Geometry: final body of the model. Coordinates: model frame, mm. A direction names the side the tool comes from. Give positions to 0.01 mm unless a question says otherwise; leave off trailing zeros. Order: outer loops, then holes, each group sorted by start corner. A loop starts at its lowest first (then second) coordinate and runs counter-clockwise, first axis right, second up. Notation, with made-up numbers: (26.25, 21) -> (50.25, 21) arc R35 cw to (50.25, 57) -> close; hole circle Ø8 at (-11, -34.75). An arc over 180 degrees is marked (long way). Write item = value, one per line.
```python
from build123d import *

# Parameters (mm, degrees)
CYLINDER049_R           = 0.8
CYLINDER049_DEPTH       = 10
CYLINDER048_R           = 0.8
CYLINDER048_DEPTH       = 10
CYLINDER017_R           = 1
CYLINDER017_DEPTH       = 10
CYLINDER017_ROLL_ANGLE  = 90
CYLINDER011_R           = 2
CYLINDER011_DEPTH       = 10
CYLINDER011_PITCH_ANGLE = 90
CYLINDER014_R           = 2
CYLINDER014_DEPTH       = 10
CYLINDER014_PITCH_ANGLE = 90
CYLINDER013_R           = 2
CYLINDER013_DEPTH       = 10
CYLINDER013_PITCH_ANGLE = 90
CYLINDER015_R           = 2
CYLINDER015_DEPTH       = 10
CYLINDER015_PITCH_ANGLE = 90
CYLINDER002_W           = 14
CYLINDER002_H           = 8
CYLINDER002_ANGLE       = 180
CYLINDER001_W           = 15
CYLINDER001_H           = 10
CYLINDER001_ANGLE       = 180
CYLINDER003_W           = 14
CYLINDER003_H           = 8
CYLINDER003_ANGLE       = 180
CYLINDER_W              = 15
CYLINDER_H              = 10
CYLINDER_ANGLE          = 180
BOX001_W                = 28
BOX001_H                = 21
BOX001_DEPTH            = 8
BOX_W                   = 30
BOX_H                   = 21
BOX_DEPTH               = 10
FUSION_PLACEMENT_ANGLE  = 180
BOX014_W                = 28
BOX014_H                = 3
BOX014_DEPTH            = 3
BOX007_W                = 30
BOX007_H                = 3
BOX007_DEPTH            = 1


with BuildPart() as cilindro049:
    # Cylinder049 → Cylinder049 (new body)
    with BuildSketch(Plane(origin=(11, -17, -15), x_dir=(1, 0, 0), z_dir=(0, 0, 1))):
        Circle(CYLINDER049_R)
    extrude(amount=CYLINDER049_DEPTH)


with BuildPart() as cilindro048:
    # Cylinder048 → Cylinder048 (new body)
    with BuildSketch(Plane(origin=(11, -4, -15), x_dir=(1, 0, 0), z_dir=(0, 0, 1))):
        Circle(CYLINDER048_R)
    extrude(amount=CYLINDER048_DEPTH)


with BuildPart() as cilindro017:
    # Cylinder017 → Cylinder017 (new body)
    with BuildSketch(Plane.XY):
        Circle(CYLINDER017_R)
    extrude(amount=CYLINDER017_DEPTH)


with BuildPart() as cilindro017_1:
    # Cylinder017 roll: moved
    add(cilindro017.part.rotate(Axis((0, 0, 0), (1, 0, 0)), CYLINDER017_ROLL_ANGLE))


with BuildPart() as cilindro017_2:
    # Cylinder017 placement: moved
    add(cilindro017_1.part.moved(Location((-14, 90, 38.5))))


with BuildPart() as cilindro011:
    # Cylinder011 → Cylinder011 (new body)
    with BuildSketch(Plane.XY):
        Circle(CYLINDER011_R)
    extrude(amount=CYLINDER011_DEPTH)


with BuildPart() as cilindro011_1:
    # Cylinder011 pitch: moved
    add(cilindro011.part.rotate(Axis((0, 0, 0), (0, 1, 0)), CYLINDER011_PITCH_ANGLE))


with BuildPart() as cilindro011_2:
    # Cylinder011 placement: moved
    add(cilindro011_1.part.moved(Location((-32, 72.5, 39.5))))


with BuildPart() as cilindro014:
    # Cylinder014 → Cylinder014 (new body)
    with BuildSketch(Plane.XY):
        Circle(CYLINDER014_R)
    extrude(amount=CYLINDER014_DEPTH)


with BuildPart() as cilindro014_1:
    # Cylinder014 pitch: moved
    add(cilindro014.part.rotate(Axis((0, 0, 0), (0, 1, 0)), CYLINDER014_PITCH_ANGLE))


with BuildPart() as cilindro014_2:
    # Cylinder014 placement: moved
    add(cilindro014_1.part.moved(Location((-5, 46.5, 39.5))))


with BuildPart() as cilindro013:
    # Cylinder013 → Cylinder013 (new body)
    with BuildSketch(Plane.XY):
        Circle(CYLINDER013_R)
    extrude(amount=CYLINDER013_DEPTH)


with BuildPart() as cilindro013_1:
    # Cylinder013 pitch: moved
    add(cilindro013.part.rotate(Axis((0, 0, 0), (0, 1, 0)), CYLINDER013_PITCH_ANGLE))


with BuildPart() as cilindro013_2:
    # Cylinder013 placement: moved
    add(cilindro013_1.part.moved(Location((-32, 46.5, 39.5))))


with BuildPart() as cilindro015:
    # Cylinder015 → Cylinder015 (new body)
    with BuildSketch(Plane.XY):
        Circle(CYLINDER015_R)
    extrude(amount=CYLINDER015_DEPTH)


with BuildPart() as cilindro015_1:
    # Cylinder015 pitch: moved
    add(cilindro015.part.rotate(Axis((0, 0, 0), (0, 1, 0)), CYLINDER015_PITCH_ANGLE))


with BuildPart() as cilindro015_2:
    # Cylinder015 placement: moved
    add(cilindro015_1.part.moved(Location((-5, 72.5, 39.5))))


with BuildPart() as cilindro002:
    # Cylinder002 → Cylinder002 (revolve)
    with BuildSketch(Plane(origin=(16, 49, -36), x_dir=(1, 0, 0), z_dir=(0, 1, 0))):
        with Locations((7, 4)):
            Rectangle(CYLINDER002_W, CYLINDER002_H)
    revolve(axis=Axis((16, 49, -36), (0, 0, -1)), revolution_arc=CYLINDER002_ANGLE)


with BuildPart() as cut001:
    # Cylinder001 → Cylinder001 (revolve)
    with BuildSketch(Plane(origin=(16, 49, -34), x_dir=(1, 0, 0), z_dir=(0, 1, 0))):
        with Locations((7.5, 5)):
            Rectangle(CYLINDER001_W, CYLINDER001_H)
    revolve(axis=Axis((16, 49, -34), (0, 0, -1)), revolution_arc=CYLINDER001_ANGLE)

    # Cut001: cut Cilindro002
    add(cilindro002.part, mode=Mode.SUBTRACT)


with BuildPart() as cut001_1:
    # Cut001 placement: moved
    add(cut001.part.moved(Location((-3, 0, 0))))


with BuildPart() as cilindro003:
    # Cylinder003 → Cylinder003 (revolve)
    with BuildSketch(Plane(origin=(13, 70, -36), x_dir=(-1, 0, 0), z_dir=(0, -1, 0))):
        with Locations((7, 4)):
            Rectangle(CYLINDER003_W, CYLINDER003_H)
    revolve(axis=Axis((13, 70, -36), (0, 0, -1)), revolution_arc=CYLINDER003_ANGLE)


with BuildPart() as cut002:
    # Cylinder → Cylinder (revolve)
    with BuildSketch(Plane(origin=(13, 70, -34), x_dir=(-1, 0, 0), z_dir=(0, -1, 0))):
        with Locations((7.5, 5)):
            Rectangle(CYLINDER_W, CYLINDER_H)
    revolve(axis=Axis((13, 70, -34), (0, 0, -1)), revolution_arc=CYLINDER_ANGLE)

    # Cut002: cut Cilindro003
    add(cilindro003.part, mode=Mode.SUBTRACT)


with BuildPart() as cubo001:
    # Box001 → Box001 (new body)
    with BuildSketch(Plane(origin=(-1, 49, -44), x_dir=(1, 0, 0), z_dir=(0, 0, 1))):
        with Locations((14, 10.5)):
            Rectangle(BOX001_W, BOX001_H)
    extrude(amount=BOX001_DEPTH)


with BuildPart() as cut025:
    # Box → Box (new body)
    with BuildSketch(Plane(origin=(-2, 49, -44), x_dir=(1, 0, 0), z_dir=(0, 0, 1))):
        with Locations((15, 10.5)):
            Rectangle(BOX_W, BOX_H)
    extrude(amount=BOX_DEPTH)

    # Cut: cut Cubo001
    add(cubo001.part, mode=Mode.SUBTRACT)

    # Fusion: union Cut001, Cut002
    add(cut001_1.part)
    add(cut002.part)


with BuildPart() as cut025_1:
    # Fusion placement: moved
    add(cut025.part.rotate(Axis((0, 0, 0), (0, 1, 0)), FUSION_PLACEMENT_ANGLE))

    # Cut021: cut Cilindro015
    add(cilindro015_2.part, mode=Mode.SUBTRACT)

    # Cut022: cut Cilindro013
    add(cilindro013_2.part, mode=Mode.SUBTRACT)

    # Cut023: cut Cilindro014
    add(cilindro014_2.part, mode=Mode.SUBTRACT)

    # Cut024: cut Cilindro011
    add(cilindro011_2.part, mode=Mode.SUBTRACT)

    # Cut025: cut Cilindro017
    add(cilindro017_2.part, mode=Mode.SUBTRACT)


with BuildPart() as cubo014:
    # Box014 → Box014 (new body)
    with BuildSketch(Plane(origin=(-27, 58, 41), x_dir=(1, 0, 0), z_dir=(0, 0, 1))):
        with Locations((14, 1.5)):
            Rectangle(BOX014_W, BOX014_H)
    extrude(amount=BOX014_DEPTH)


with BuildPart() as cut068:
    # Box007 → Box007 (new body)
    with BuildSketch(Plane(origin=(-28, 58, 44), x_dir=(1, 0, 0), z_dir=(0, 0, 1))):
        with Locations((15, 1.5)):
            Rectangle(BOX007_W, BOX007_H)
    extrude(amount=BOX007_DEPTH)

    # Fusion002010: union Cubo014
    add(cubo014.part)

    # Fusion002015: union Cut025
    add(cut025_1.part)


with BuildPart() as cut068_1:
    # Fusion002015 placement: moved
    add(cut068.part.moved(Location((13, -70, -44))))

    # Cut067: cut Cilindro048
    add(cilindro048.part, mode=Mode.SUBTRACT)

    # Cut068: cut Cilindro049
    add(cilindro049.part, mode=Mode.SUBTRACT)


solid = cut068_1.part
```
1) Reachability of faces 4 (the face through (0, -10, -8)), 5 (the face through (-14.137, -25.452, -4.066)), 6 (the face through (3, -35, 0)), 7 (the face through (0, -12, -1)), 8 (the face through (-1.13, 14.44, -4.51)) from +Z, -Z, +X, -X, +Y, -Y: full face, straight path, thin tool, end or side. Return the list, or none.
Check sheet entries:
face_4 = none
face_5 = +X, -X
face_6 = +Z, +X, -X, -Y
face_7 = +Z
face_8 = +Y
2) Section query C-C (x = -10). Output: boundary loops of the cut face in (y, z).
Check sheet entries:
outline = (-32.18, -10) -> (11.18, -10) -> (11.18, 0) -> (9.8, 0) -> (9.8, -8) -> (-30.8, -8) -> (-30.8, 0) -> (-32.18, 0) -> close; (-12, -3) -> (-9, -3) -> (-9, 1) -> (-12, 1) -> close
3) Line query: line 1 (X direction, y = -1.5, z = -6.75); line 2 (Y direction, x = -12, z = -0.25); line 3 (Z direction, x = 14.5, y = 2.5). Output: solid intervals per line, ascending. Write a range as from..to.
Check sheet entries:
line_1 = -15..-14, 14..15
line_2 = -30..-28.21, -12..-9, 7.21..9
line_3 = -10..-6.5, -2.5..0
4) Section query B-B (z = -7.25). Output: boundary loops of the cut face in (x, y), plus the area to 3 significant figures.
Check sheet entries:
outline = (-15, -21) arc R15 ccw to (15, -21) -> (15, 0) arc R15 ccw to (-15, 0) -> close; hole (-14, -21) arc R14 ccw to (14, -21) -> (14, 0) arc R14 ccw to (-14, 0) -> close
area = 133 mm²
5) First-contact query: P1, Ø2, axis at x = -11.5, z = -5.5, coming from the +Y side; P2, Ø2, axis at x = 11, y = -17, coming from the +Z side; P3, Ø2, axis at x = 3, z = -0.5, coming from the -Y side. Flat tips, straight axial feed; report the tip coordinate or a pass-through.
Check sheet entries:
P1 = 10.71
P2 = -8
P3 = -35.87
6) Mould query, pull axis X, two halves, no side actions, for faces 1 (the face through (0, -36, -5)), 2 (the face through (11.37, -4.71, -9.01)), 3 (the face through (0, -10, 1)). Classes: +X half, -X half, draft (parallel to the pull), parting line (faces both ways), or undercut.
Check sheet entries:
face_1 = parting line
face_2 = undercut
face_3 = draft
7) Section query D-D (z = -0.75). Output: boundary loops of the cut face in (x, y), plus the area to 3 significant figures.
Check sheet entries:
outline = (-15, -21) arc R15 ccw to (15, -21) -> (15, 0) arc R15 ccw to (-15, 0) -> close; hole (-14, -21) arc R14 ccw to (14, -21) -> (14, -12) -> (-14, -12) -> close; hole (-14, -9) -> (14, -9) -> (14, 0) arc R14 ccw to (-14, 0) -> close
area = 217 mm²
8) Section query A-A (y = -4). Output: boundary loops of the cut face in (x, z).
Check sheet entries:
outline = (-15, -10) -> (10.2, -10) -> (10.2, -8) -> (-14, -8) -> (-14, 0) -> (-15, 0) -> close; (11.8, -10) -> (15, -10) -> (15, 0) -> (14, 0) -> (14, -8) -> (11.8, -8) -> close
